```python
from build123d import *

# Parameters (mm, degrees)
F1_DEPTH = 25.4
F2_R     = 12.7
F3_DEPTH = 19.05
F4_R     = 19.05
F2_R_2   = 3.175
F5_DEPTH = 25.4
F6_R     = 6.35
F7_DEPTH = 6.35


with BuildPart() as f1:
    # F0 (on Top) → F1 (new body)
    with BuildSketch(Plane.XY):
        with BuildLine():
            Line((88.281516, 60.815624), (0, 60.815624))
            ThreePointArc((0, 60.815624), (-60.815624, 0), (0, -60.815624))
            Line((0, -60.815624), (88.281516, -60.815624))
            Line((88.281516, -60.815624), (88.281516, 60.815624))
        make_face()
    extrude(amount=F1_DEPTH)

    # F2 (on face) → F3 (cut)
    with BuildSketch(Plane.XY.offset(25.4)):
        with BuildLine():
            Line((88.281516, 46.0375), (21.475302, 46.0375))
            ThreePointArc((21.475302, 46.0375), (-50.8, 0), (21.475302, -46.0375))
            Line((21.475302, -46.0375), (88.281516, -46.0375))
            Line((88.281516, -46.0375), (88.281516, -31.75))
            Line((88.281516, -31.75), (39.655737, -31.75))
            ThreePointArc((39.655737, -31.75), (50.8, 0), (39.655737, 31.75))
            Line((39.655737, 31.75), (88.281516, 31.75))
            Line((88.281516, 31.75), (88.281516, 46.0375))
        make_face()
        Circle(F2_R, mode=Mode.SUBTRACT)
    extrude(amount=-F3_DEPTH, mode=Mode.SUBTRACT)

    # F4
    f4_edges = [f1.edges().sort_by_distance(p)[0] for p in [
        (21.475302, 46.0375, 15.875),
        (21.475302, -46.0375, 15.875),
    ]]
    fillet(f4_edges, radius=F4_R)

    # F2 (on face) → F5 (cut)
    with BuildSketch(Plane.XY.offset(25.4)):
        Circle(F2_R_2)
    extrude(amount=-F5_DEPTH, mode=Mode.SUBTRACT)

    # F6 (on face) → F7 (cut)
    with BuildSketch(Plane(origin=(0, 0, 0), x_dir=(1, 0, 0), z_dir=(0, 0, -1))):
        Circle(F6_R)
    extrude(amount=-F7_DEPTH, mode=Mode.SUBTRACT)


solid = f1.part
```
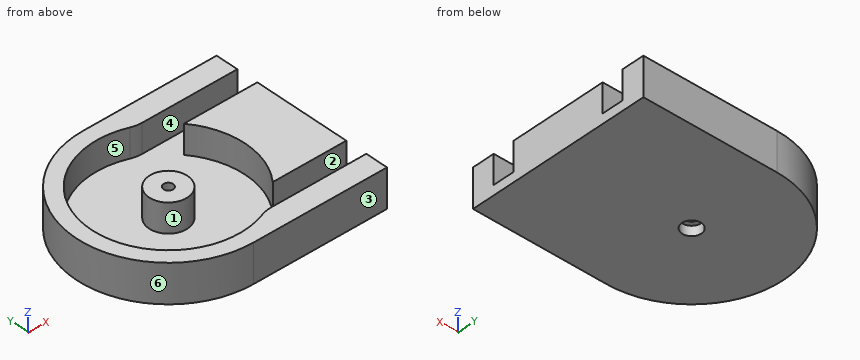
Geometry check sheet. Reference: the model listing, model coordinates, mm. Face numbers are marked on the shaded views. A direction names the side the tool comes from. Give positions to 0.01 mm unless a question says otherwise; leave off trailing zeros. Order: outer loops, then holes, each group sorted by start corner. A loop starts at its lowest first (then second) coordinate and runs counter-clockwise, first axis right, second up. Notation, with made-up numbers: (49, 86.5) - (82, 86.5) arc R20 ccw to (82, 102.5) - close; hole circle Ø11 at (4.5, 73.5). An arc over 180 degrees is marked (long way). Answer in a Markdown table with one row per item. Add a question column.
Q1. Cross-section at A-A, the plane z = 10. Count the separate pieces of the cut face and the enclosed holes in it, then the cut area to 3 significant figures.
Q2. Material ranges on probe 1 along Y at (x, z) = (0, 11) (3 decimals); probe 2 along Y at (x, z) = (38.5, 7.5); probe 3 along X at (y, z) = (0, 2.5), recorded low to high. Write a range as from..to.
Q3. Tool access check on the marked faces 1, 2 and 3. Record the directions out of +Z, -Z, +X, -X, +Y, -Y that give a thin tool (end or side, any length) a straight path to the whole face; none if there is none.
Q4. Gauge pin test, flat ends, axial feed: pin 1 (1.5 mm diameter, centred on x = -21, z = 4, fed in from -Y); pin 2 (10 mm diameter, centred on x = 0, y = 0, fed in from -Z); pin 3 (3 mm diameter, centred on x = -43.5, z = 6.5, fed in from +Y); pin 4 (14 mm diameter, centred on x = 1.5, y = -0.5, fed in from -Z). Record the tip position at first contact, or that the pin passes through.
Q5. Cross-section at B-B, the plane y = 0. Enter the section's corners in (x, z) (3 decimals), then the cut area to 3 significant figures.
Q6. Cross-section at D-D, the plane y = 21.5. Enter the section's corners in (x, z).
Q7. Mould release check, pull along X, two halves, no side actions. Record for the marked faces 4, 5 and 6: pulls with the +X half, pulls with the -X half, needs draft (parallel to the pull), parting line crosses it, or undercut.
Q8. Cross-section at C-C, the plane x = -16.5. Enter the section's corners in (y, z).
Check values:
| question | item | result |
|---|---|---|
| 1 | separate pieces | 3 |
| 1 | enclosed holes | 1 |
| 1 | area | 7,310 mm^2 |
| 2 | probe 1 | y = -60.816..-50.8, -12.7..-3.175, 3.175..12.7, 50.8..60.816 |
| 2 | probe 2 | y = -60.82..-46.04, 46.04..60.82 |
| 2 | probe 3 | x = -60.82..-6.35, 6.35..88.28 |
| 3 | face 1 | +Z |
| 3 | face 2 | +Z, +X |
| 3 | face 3 | +Z, -Z, +X, -X, -Y |
| 4 | pin 1 | stops at y = -57.35 |
| 4 | pin 2 | stops at z = 6.35 |
| 4 | pin 3 | stops at y = 43.98 |
| 4 | pin 4 | stops at z = 0 |
| 5 | outline | (-60.816, 0) - (-6.35, 0) - (-6.35, 6.35) - (-3.175, 6.35) - (-3.175, 25.4) - (-12.7, 25.4) - (-12.7, 6.35) - (-50.8, 6.35) - (-50.8, 25.4) - (-60.816, 25.4) - close; (3.175, 6.35) - (6.35, 6.35) - (6.35, 0) - (88.282, 0) - (88.282, 25.4) - (50.8, 25.4) - (50.8, 6.35) - (12.7, 6.35) - (12.7, 25.4) - (3.175, 25.4) - close |
| 5 | area | 2,130 mm^2 |
| 6 | outline | (-56.89, 0) - (88.28, 0) - (88.28, 25.4) - (46.03, 25.4) - (46.03, 6.35) - (-46.03, 6.35) - (-46.03, 25.4) - (-56.89, 25.4) - close |
| 7 | face 4 | needs draft |
| 7 | face 5 | undercut |
| 7 | face 6 | pulls with the -X half |
| 8 | outline | (-58.53, 0) - (58.53, 0) - (58.53, 25.4) - (48.05, 25.4) - (48.05, 6.35) - (-48.05, 6.35) - (-48.05, 25.4) - (-58.53, 25.4) - close |
